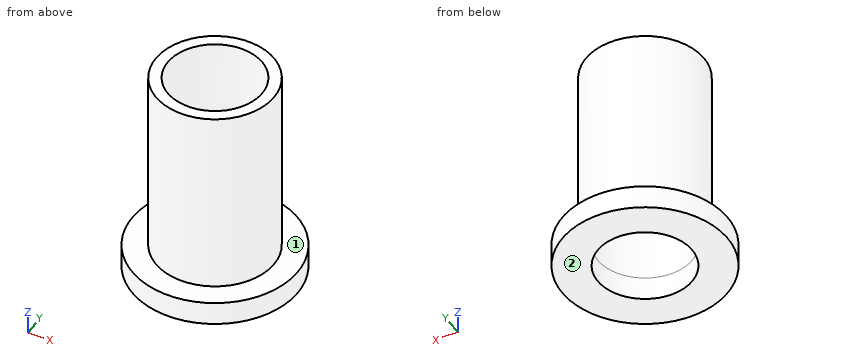
```python
from build123d import *

# Parameters (mm, degrees)
SKETCH1_R           = 7.9375
SKETCH1_R_2         = 6.35
BOSS_EXTRUDE1_DEPTH = 25.4
SKETCH2_R           = 11.1125
SKETCH2_R_2         = 6.35
BOSS_EXTRUDE2_DEPTH = 3.175


with BuildPart() as part:
    # Sketch1 → Boss-Extrude1 (new body)
    with BuildSketch(Plane.XY):
        Circle(SKETCH1_R)
        Circle(SKETCH1_R_2, mode=Mode.SUBTRACT)
    extrude(amount=BOSS_EXTRUDE1_DEPTH)

    # Sketch2 → Boss-Extrude2 (add)
    with BuildSketch(Plane(origin=(0, 0, 0), x_dir=(-1, 0, 0), z_dir=(0, 0, -1))):
        Circle(SKETCH2_R)
        Circle(SKETCH2_R_2, mode=Mode.SUBTRACT)
    extrude(amount=BOSS_EXTRUDE2_DEPTH)


solid = part.part
```
Verification items for the finished model (mm, model axes). Face numbers are marked on the shaded views. A direction names the side the tool comes from. Round coordinates to 2 decimals unless told otherwise and drop trailing zeros. Write each loop counter-clockwise with the first axis right and the second up, starting at its lowest first coordinate (ties: lowest second). Pieces come first, ordered by that corner, then holes. Notation, with made-up numbers: (12, 23.25) - (16, 23.25) arc R31 ccw to (16, 52.25) - close; hole circle Ø8 at (43, 37). An arc over 180 degrees is marked (long way). Answer as a JSON object with one key per item and string values. Group by question number.
Q1. Go/stop test with flat-tipped pins: pin 1 Ø4 at (y, z) = (7, 20) entering from -X; pin 2 Ø3 at (y, z) = (2.5, 7.5) entering from +X; pin 3 Ø1.5 at (x, z) = (1.5, 19) entering from +Y; pin 4 Ø7.5 at (x, y) = (0, 0) entering from +Z. Record where each tip stops, or that it passes through.
Q2. Thickness scan on line 1 (Y direction, x = 0, z = 12.25); line 2 (X direction, y = -0.25, z = 6.75); line 3 (Y direction, x = 0, z = -1.7). Record the ranges inside material, lowest first.
Q3. Tool access check on the marked faces 1 and 2. Record the directions out of +Z, -Z, +X, -X, +Y, -Y that give a thin tool (end or side, any length) a straight path to the whole face; none if there is none.
Q4. Section check D-D, the plane y = -6.75. Enter the section's corners in (x, z) (3 decimals), plus the area to 3 significant figures.
Found:
{
 "1": {"pin 1": "stops at x = -6.16", "pin 2": "stops at x = 7.87", "pin 3": "stops at y = 7.9", "pin 4": "passes through"},
 "2": {"line 1": "y = -7.94 to -6.35, 6.35 to 7.94", "line 2": "x = -7.93 to -6.35, 6.35 to 7.93", "line 3": "y = -11.11 to -6.35, 6.35 to 11.11"},
 "3": {"face 1": "+Z", "face 2": "-Z, +X, -X, +Y, -Y"},
 "4": {"outline": "(-8.828, -3.175) - (8.828, -3.175) - (8.828, 0) - (4.176, 0) - (4.176, 25.4) - (-4.176, 25.4) - (-4.176, 0) - (-8.828, 0) - close", "area": "268 mm^2"}
}
